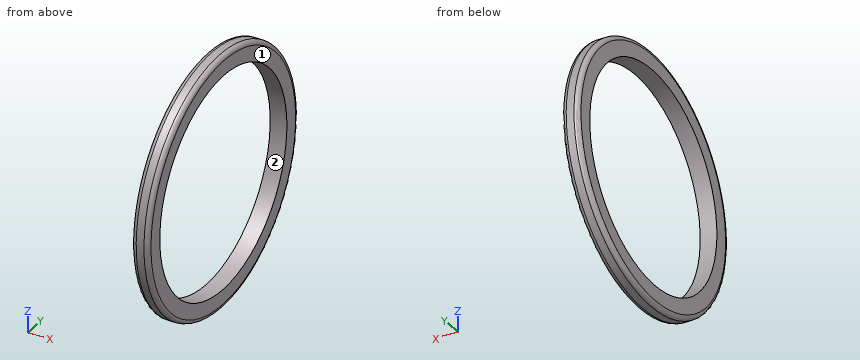
```python
from build123d import *

# Parameters (mm, degrees)
SKETCH1_R           = 230
BOSS_EXTRUDE1_DEPTH = 30
FILLET1_R           = 8
SKETCH2_R           = 195
CUT_EXTRUDE1_DEPTH  = 327.649659421


with BuildPart() as part:
    # Sketch1 → Boss-Extrude1 (new body)
    with BuildSketch(Plane(origin=(0, 0, 0), x_dir=(0, 0, -1), z_dir=(1, 0, 0))):
        Circle(SKETCH1_R)
    extrude(amount=BOSS_EXTRUDE1_DEPTH)

    # Fillet1
    fillet1_edges = [part.edges().sort_by_distance(p)[0] for p in [
        (0, 0, 230),
        (30, 0, 230),
    ]]
    fillet(fillet1_edges, radius=FILLET1_R)

    # Sketch2 → Cut-Extrude1 (cut, through all)
    with BuildSketch(Plane(origin=(30, 0, 0), x_dir=(0, 0, -1), z_dir=(1, 0, 0))):
        Circle(SKETCH2_R)
    extrude(amount=-CUT_EXTRUDE1_DEPTH, mode=Mode.SUBTRACT)


solid = part.part
```
For this review, take the finished solid that the model builds, in its own axes (mm). Face numbers are marked on the shaded views. Round coordinates to 2 decimals unless told otherwise and drop trailing zeros. Loops run counter-clockwise (first coordinate to the right, second up) from the corner with the lowest first, then second, coordinate; pieces in that order, holes last.
(1) We need section C-C (x = 17). Give the boundary of the cut face in (y, z), plus the area to 3 significant figures.
Returned:
outline: circle Ø460 at (0, 0); hole circle Ø390 at (0, 0)
area: 46,700 mm2
(2) Clearance check with flat-ended pins moving along their axes: P1, Ø8, axis at x = 16.5, z = -49, coming from the -Y side; P2, Ø2, axis at x = 13, y = -161, coming from the +Z side; P3, Ø4, axis at x = 15, y = -34, coming from the -Z side. State where each tip first meets the part, or that it passes through.
Returned:
P1: stops at y = -225.55
P2: stops at z = 165.23
P3: stops at z = -227.76
(3) Mouldability with a two-part tool opening along Z and no side actions: class the marked faces 1 and 2 as released by +Z, released by -Z, zero draft, split by the parting line, or undercut.
Returned:
face 1: zero draft
face 2: undercut
(4) We need section A-A (z = 0). Give the boundary of the cut face in (x, y), plus the area to 3 significant figures.
Returned:
outline: (0, -222) arc R8 ccw to (8, -230) - (22, -230) arc R8 ccw to (30, -222) - (30, -195) - (0, -195) - close; (0, 195) - (30, 195) - (30, 222) arc R8 ccw to (22, 230) - (8, 230) arc R8 ccw to (0, 222) - close
area: 2,050 mm2
(5) Wall thickness on line 1 along Y through (x, z) = (23.25, 0); line 2 along Y through (x, z) = (15.25, 0); line 3 along Z through (x, y) = (11, 156.5): over which ranges is each line inside the solid? List them lowest first.
Returned:
line 1: y = -229.9 to -195, 195 to 229.9
line 2: y = -230 to -195, 195 to 230
line 3: z = -168.55 to -116.33, 116.33 to 168.55
